Here's how the part is built. I have some questions about the finished solid (model axes, mm). A direction names the side the tool comes from. Coordinates: 2 decimals unless noted, no trailing zeros. Write each loop counter-clockwise with the first axis right and the second up, starting at its lowest first coordinate (ties: lowest second). Pieces come first, ordered by that corner, then holes.
Item 1: If we section it at B-B (z = 6.75): Please give me the cut outline in (x, y), then the cut area to 3 significant figures.
Item 2: If we section it at D-D (y = 7): Please give me the cut outline in (x, z).
Item 3: If I drill on line 1 (X direction, y = 30, z = 9.5); line 2 (Y direction, x = 59.5, z = 14.25); line 3 (Z direction, x = 250, y = 3), over which ranges is the centre line in solid material (lowest first)?
Item 4: For faces 1 (the face through (22, 30, 9)), 2 (the face through (171, 19, 18)), 3 (the face through (170, 8, 0)), which set-ups out of +Z, -Z, +X, -X, +Y, -Y let a thin tool reach every point of the face, with its end or its side?
Item 5: If we section it at A-A (y = 34.5): Please give me the cut outline in (x, z), then the cut area to 3 significant figures.
Item 6: I'm going to push flat-ended pins straight in: pin 1 Ø2 at (x, y) = (200, 6) entering from +Z; pin 2 Ø8.5 at (x, z) = (157, 12) entering from -Y; pin 3 Ø5 at (y, z) = (32.5, 12.5) entering from -X. Where does each tip first touch, or does it pass through?
Item 7: If we section it at C-C (x = 141.5): Please give me the cut outline in (y, z), then the cut area to 3 significant figures.
Item 8: We'd pull the mould along X, two halves only. Please class faces 4 (the face through (322.2, 30, 10)), 5 (the face through (174, 18, 10)), 6 (the face through (20, 29, 9)): +X half, -X half, draft (parallel to the pull), parting line (faces both ways), or undercut.
from build123d import *

# Parameters (mm, degrees)
SKETCH_1_W                       = 2
SKETCH_1_H                       = 20
EXTRUDE_1_DEPTH                  = 344.2
SM_EDGE_FLANGE_1_STRIP_W         = 10
SM_EDGE_FLANGE_1_STRIP_H         = 2
SM_EDGE_FLANGE_1_STRIP_CUT_DEPTH = 344.2
SM_EDGE_FLANGE_1_DEPTH           = 344.2
SM_EDGE_FLANGE_2_STRIP_W         = 30
SM_EDGE_FLANGE_2_STRIP_H         = 2
SM_EDGE_FLANGE_2_STRIP_CUT_DEPTH = 17
SM_EDGE_FLANGE_2_DEPTH           = 17
SM_EDGE_FLANGE_3_STRIP_W         = 30
SM_EDGE_FLANGE_3_STRIP_H         = 2
SM_EDGE_FLANGE_3_STRIP_CUT_DEPTH = 17
SM_EDGE_FLANGE_3_DEPTH           = 17


# Sheet-metal steps are written as plain solids
with BuildPart() as part:
    # Sketch 1 → Бобышка-Вытянуть1 (new body)
    with BuildSketch(Plane(origin=(0, 0, 0), x_dir=(0, 0, -1), z_dir=(1, 0, 0))):
        with Locations((1, 10)):
            Rectangle(SKETCH_1_W, SKETCH_1_H)
    extrude(amount=EXTRUDE_1_DEPTH)

    # Ребро-кромка1 strip (across the edge) → Ребро-кромка1 strip cut (cut)
    with BuildSketch(Plane(origin=(344.2, 20, 0), x_dir=(0, -1, 0), z_dir=(-1, 0, 0))):
        with Locations((-2, -1)):
            Rectangle(SM_EDGE_FLANGE_1_STRIP_W, SM_EDGE_FLANGE_1_STRIP_H)
    extrude(amount=SM_EDGE_FLANGE_1_STRIP_CUT_DEPTH, mode=Mode.SUBTRACT)

    # Ребро-кромка1 section (across the edge) → Ребро-кромка1 (add)
    with BuildSketch(Plane(origin=(344.2, 20, 0), x_dir=(0, -1, 0), z_dir=(-1, 0, 0))):
        with BuildLine():
            Line((0, 1), (0, 18))
            Line((0, 18), (2, 18))
            Line((2, 18), (2, 1))
            ThreePointArc((2, 1), (2.292893219, 0.292893219), (3, 0))
            Line((3, 0), (3, -2))
            ThreePointArc((3, -2), (0.878679656, -1.121320344), (0, 1))
        make_face()
    extrude(amount=SM_EDGE_FLANGE_1_DEPTH)

    # Ребро-кромка2 strip (across the edge) → Ребро-кромка2 strip cut (cut)
    with BuildSketch(Plane(origin=(20, 20, 1), x_dir=(1, 0, 0), z_dir=(0, 0, 1))):
        with Locations((-12, -1)):
            Rectangle(SM_EDGE_FLANGE_2_STRIP_W, SM_EDGE_FLANGE_2_STRIP_H)
    extrude(amount=SM_EDGE_FLANGE_2_STRIP_CUT_DEPTH, mode=Mode.SUBTRACT)

    # Ребро-кромка2 section (across the edge) → Ребро-кромка2 (add)
    with BuildSketch(Plane(origin=(20, 20, 1), x_dir=(1, 0, 0), z_dir=(0, 0, 1))):
        with BuildLine():
            Line((0, 1), (0, 18))
            Line((0, 18), (2, 18))
            Line((2, 18), (2, 1))
            ThreePointArc((2, 1), (2.292893219, 0.292893219), (3, 0))
            Line((3, 0), (3, -2))
            ThreePointArc((3, -2), (0.878679656, -1.121320344), (0, 1))
        make_face()
    extrude(amount=SM_EDGE_FLANGE_2_DEPTH)

    # Ребро-кромка3 strip (across the edge) → Ребро-кромка3 strip cut (cut)
    with BuildSketch(Plane(origin=(324.2, 20, 18), x_dir=(-1, 0, 0), z_dir=(0, 0, -1))):
        with Locations((-12, -1)):
            Rectangle(SM_EDGE_FLANGE_3_STRIP_W, SM_EDGE_FLANGE_3_STRIP_H)
    extrude(amount=SM_EDGE_FLANGE_3_STRIP_CUT_DEPTH, mode=Mode.SUBTRACT)

    # Ребро-кромка3 section (across the edge) → Ребро-кромка3 (add)
    with BuildSketch(Plane(origin=(324.2, 20, 18), x_dir=(-1, 0, 0), z_dir=(0, 0, -1))):
        with BuildLine():
            Line((0, 1), (0, 18))
            Line((0, 18), (2, 18))
            Line((2, 18), (2, 1))
            ThreePointArc((2, 1), (2.292893219, 0.292893219), (3, 0))
            Line((3, 0), (3, -2))
            ThreePointArc((3, -2), (0.878679656, -1.121320344), (0, 1))
        make_face()
    extrude(amount=SM_EDGE_FLANGE_3_DEPTH)


solid = part.part
Answer list:
1. outline: (20, 21) arc R3 ccw to (23, 18) - (321.2, 18) arc R3 ccw to (324.2, 21) - (324.2, 38) - (322.2, 38) - (322.2, 21) arc R1 cw to (321.2, 20) - (23, 20) arc R1 cw to (22, 21) - (22, 38) - (20, 38) - close
1. area: 677 mm2
2. outline: (0, -2) - (344.2, -2) - (344.2, 0) - (0, 0) - close
3. line 1: x = 20 to 22, 322.2 to 324.2
3. line 2: y = 18 to 20
3. line 3: z = -2 to 0
4. face 1: +Z, -Z, +Y
4. face 2: +Z, +X, -X, +Y, -Y
4. face 3: +Z, +X, -X, -Y
5. outline: (20, 1) - (22, 1) - (22, 18) - (20, 18) - close; (322.2, 1) - (324.2, 1) - (324.2, 18) - (322.2, 18) - close
5. area: 68.0 mm2
6. pin 1: stops at z = 0
6. pin 2: stops at y = 18
6. pin 3: stops at x = 20
7. outline: (0, -2) - (17, -2) arc R3 ccw to (20, 1) - (20, 18) - (18, 18) - (18, 1) arc R1 cw to (17, 0) - (0, 0) - close
7. area: 74.3 mm2
8. face 4: undercut
8. face 5: draft
8. face 6: -X half
